from build123d import *

# Parameters (mm, degrees)
SKETCH_1_R      = 40
SKETCH_1_R_2    = 12.5
SKETCH_1_R_3    = 2
SKETCH_1_R_4    = 3
EXTRUDE_1_DEPTH = 10


with BuildPart() as part:
    # 草图1 → 凸台-拉伸1 (new body)
    with BuildSketch(Plane.XY):
        with Locations((-35.478977731, 11.880589307)):
            Circle(SKETCH_1_R)
        with Locations((-35.478977731, 11.880589307)):
            Circle(SKETCH_1_R_2, mode=Mode.SUBTRACT)
        with Locations((-35.478977731, 29.130589307)):
            Circle(SKETCH_1_R_3, mode=Mode.SUBTRACT)
        with Locations((-20.540039516, 20.505589307)):
            Circle(SKETCH_1_R_3, mode=Mode.SUBTRACT)
        with Locations((-20.540039516, 3.255589307)):
            Circle(SKETCH_1_R_3, mode=Mode.SUBTRACT)
        with Locations((-35.478977731, -5.369410693)):
            Circle(SKETCH_1_R_3, mode=Mode.SUBTRACT)
        with Locations((-50.417915947, 3.255589307)):
            Circle(SKETCH_1_R_3, mode=Mode.SUBTRACT)
        with Locations((-50.417915947, 20.505589307)):
            Circle(SKETCH_1_R_3, mode=Mode.SUBTRACT)
        with Locations((-35.478977731, 46.880589307)):
            Circle(SKETCH_1_R_4, mode=Mode.SUBTRACT)
    extrude(amount=EXTRUDE_1_DEPTH)


solid = part.part
Verification items for the finished model (mm, model axes). Give positions to 0.01 mm unless a question says otherwise; leave off trailing zeros. Write each loop counter-clockwise with the first axis right and the second up, starting at its lowest first coordinate (ties: lowest second). Pieces come first, ordered by that corner, then holes.
(1) Cross-section at B-B (z = 9). State how many separate pieces and enclosed holes the cut face has, plus the area to 3 significant figures.
(2) Mould release check, pull along Y, two halves, no side actions. Record for faces 1 (the face through (-23.556, 15.635, 4.93)), 2 (the face through (-33.631, 28.365, 4.93)), 3 (the face through (2.674, 23.896, 4.93)), 4 (the face through (-45, 21, 0)): +Y half, -Y half, draft (parallel to the pull), parting line (faces both ways), or undercut.
(3) Cross-section at A-A (x = -39.5). Enter the section's corners in (y, z) (3 decimals), plus the area to 3 significant figures.
(4) Material ranges on line 1 (Y direction, x = -21.5, z = 2.5); line 2 (X direction, y = 20, z = 5.5) (3 decimals); line 3 (Y direction, x = -20, z = 4.25), recorded low to high.
(5) Cross-section at D-D (x = -19.5). Enter the section's corners in (y, z).
(6) Gauge pin test, flat ends, axial feed: pin 1 (3 mm diameter, centred on x = -35.48, y = -5.37, fed in from +Z); pin 2 (1 mm diameter, centred on y = -12.5, z = 4, fed in from +X); pin 3 (1.5 mm diameter, centred on x = -64.5, z = 8, fed in from +Y); pin 4 (1 mm diameter, centred on x = -27, z = 5, fed in from -Y). Record the tip position at first contact, or that the pin passes through.
(7) Cross-section at C-C (y = 8.5). Enter the section's corners in (x, z).
Worked out:
1. separate pieces: 1
1. enclosed holes: 8
1. area: 4,430 mm2
2. face 1: undercut
2. face 2: undercut
2. face 3: parting line
2. face 4: draft
3. outline: (-27.917, 0) - (0.045, 0) - (0.045, 10) - (-27.917, 10) - close; (23.716, 0) - (51.678, 0) - (51.678, 10) - (23.716, 10) - close
3. area: 559 mm2
4. line 1: y = -25.6 to 1.5, 5.01 to 18.75, 22.26 to 49.36
4. line 2: x = -74.646 to -52.353, -48.483 to -44.983, -25.975 to -22.475, -18.605 to 3.688
4. line 3: y = -25 to 1.33, 5.18 to 18.58, 22.43 to 48.76
5. outline: (-24.79, 0) - (1.55, 0) - (1.55, 10) - (-24.79, 10) - close; (4.96, 0) - (18.8, 0) - (18.8, 10) - (4.96, 10) - close; (22.21, 0) - (48.55, 0) - (48.55, 10) - (22.21, 10) - close
6. pin 1: passes through
6. pin 2: stops at x = -3.39
6. pin 3: stops at y = 40.18
6. pin 4: stops at y = -27.32
7. outline: (-75.34, 0) - (-47.51, 0) - (-47.51, 10) - (-75.34, 10) - close; (-23.44, 0) - (4.38, 0) - (4.38, 10) - (-23.44, 10) - close
